```python
from build123d import *

# Parameters (mm, degrees)
MODEL_R             = 2.75
MODEL_R_2           = 1.524
MODEL_R_3           = 3.57
MODEL_R_4           = 3
MODEL_R_5           = 1.75
MODEL_R_6           = 2.988685284
MODEL_R_7           = 11.25
MODEL_W             = 18.00197115
MODEL_H             = 6.02504647
MODEL_W_2           = 25.001971156
MODEL_H_2           = 6.025046469
BOSS_EXTRUDE2_DEPTH = 3


with BuildPart() as part:
    # Model → Boss-Extrude2 (new body)
    with BuildSketch(Plane.XY):
        with BuildLine():
            Line((-1558.170802496, 1596.031612088), (-1558.170802496, 1743.759047656))
            ThreePointArc((-1558.170802496, 1743.759047656), (-1559.633113999, 1747.298520787), (-1563.170804742, 1748.765139071))
            Line((-1563.170804742, 1748.765139071), (-1643.16842822, 1748.765139071))
            ThreePointArc((-1643.16842822, 1748.765139071), (-1646.706118961, 1747.298520788), (-1648.168430466, 1743.759047658))
            Line((-1648.168430466, 1743.759047658), (-1648.168430466, 1596.031606131))
            ThreePointArc((-1648.168430466, 1596.031606131), (-1646.703964372, 1592.496072226), (-1643.168430466, 1591.031606131))
            Line((-1643.168430466, 1591.031606131), (-1563.170808452, 1591.031606131))
            ThreePointArc((-1563.170808452, 1591.031606131), (-1559.63526859, 1592.496072225), (-1558.170802496, 1596.031612088))
        make_face()
        with Locations((-1573.06309524, 1605.466177477)):
            Circle(MODEL_R, mode=Mode.SUBTRACT)
        with Locations((-1573.06309524, 1625.466177477)):
            Circle(MODEL_R, mode=Mode.SUBTRACT)
        with Locations((-1633.276137722, 1605.466177477)):
            Circle(MODEL_R, mode=Mode.SUBTRACT)
        with Locations((-1633.276137722, 1625.466177477)):
            Circle(MODEL_R, mode=Mode.SUBTRACT)
        with Locations((-1564.034669062, 1605.466177486)):
            Circle(MODEL_R, mode=Mode.SUBTRACT)
        with Locations((-1642.166137722, 1605.466177477)):
            Circle(MODEL_R, mode=Mode.SUBTRACT)
        with Locations((-1564.034669062, 1625.466177486)):
            Circle(MODEL_R, mode=Mode.SUBTRACT)
        with Locations((-1642.166137722, 1625.466177477)):
            Circle(MODEL_R, mode=Mode.SUBTRACT)
        with Locations((-1564.0520997, 1593.809639733)):
            Circle(MODEL_R_2, mode=Mode.SUBTRACT)
        with Locations((-1584.028829584, 1602.080803539)):
            Circle(MODEL_R_2, mode=Mode.SUBTRACT)
        with Locations((-1642.287133262, 1593.809639733)):
            Circle(MODEL_R_2, mode=Mode.SUBTRACT)
        with Locations((-1622.310403377, 1602.080803539)):
            Circle(MODEL_R_2, mode=Mode.SUBTRACT)
        with Locations((-1564.034669062, 1679.892967716)):
            Circle(MODEL_R, mode=Mode.SUBTRACT)
        with Locations((-1564.034669062, 1659.936167716)):
            Circle(MODEL_R, mode=Mode.SUBTRACT)
        with Locations((-1642.166137722, 1679.892967726)):
            Circle(MODEL_R, mode=Mode.SUBTRACT)
        with Locations((-1642.166137722, 1659.936167726)):
            Circle(MODEL_R, mode=Mode.SUBTRACT)
        with Locations((-1633.028888044, 1669.901183151)):
            Circle(MODEL_R_3, mode=Mode.SUBTRACT)
        with Locations((-1633.027603994, 1699.99200382)):
            Circle(MODEL_R_3, mode=Mode.SUBTRACT)
        with Locations((-1633.027603994, 1639.99200382)):
            Circle(MODEL_R_3, mode=Mode.SUBTRACT)
        with Locations((-1642.168430466, 1643.881204835)):
            Circle(MODEL_R_3, mode=Mode.SUBTRACT)
        with Locations((-1642.168430466, 1696.860624835)):
            Circle(MODEL_R_3, mode=Mode.SUBTRACT)
        with Locations((-1564.170802496, 1643.881204835)):
            Circle(MODEL_R_3, mode=Mode.SUBTRACT)
        with Locations((-1573.17191871, 1669.901183151)):
            Circle(MODEL_R_3, mode=Mode.SUBTRACT)
        with Locations((-1613.166137692, 1674.864567716)):
            Circle(MODEL_R, mode=Mode.SUBTRACT)
        with Locations((-1593.100403377, 1674.880803539)):
            Circle(MODEL_R, mode=Mode.SUBTRACT)
        with Locations((-1613.077133262, 1602.064639733)):
            Circle(MODEL_R_4, mode=Mode.SUBTRACT)
        with Locations((-1593.100403377, 1602.080803539)):
            Circle(MODEL_R_4, mode=Mode.SUBTRACT)
        with Locations((-1564.170802496, 1696.860624835)):
            Circle(MODEL_R_3, mode=Mode.SUBTRACT)
        with Locations((-1613.166137692, 1664.864567716)):
            Circle(MODEL_R, mode=Mode.SUBTRACT)
        with Locations((-1618.57210033, 1609.927346224)):
            Circle(MODEL_R_5, mode=Mode.SUBTRACT)
        with Locations((-1618.625460969, 1640.924100772)):
            Circle(MODEL_R_5, mode=Mode.SUBTRACT)
        with Locations((-1593.100403377, 1664.880803539)):
            Circle(MODEL_R, mode=Mode.SUBTRACT)
        with Locations((-1573.17320276, 1699.99200382)):
            Circle(MODEL_R_3, mode=Mode.SUBTRACT)
        with Locations((-1623.370056938, 1685.360521432)):
            Circle(MODEL_R_4, mode=Mode.SUBTRACT)
        with Locations((-1582.81965611, 1685.466121434)):
            Circle(MODEL_R_6, mode=Mode.SUBTRACT)
        with Locations((-1623.370056938, 1625.360521432)):
            Circle(MODEL_R_4, mode=Mode.SUBTRACT)
        with Locations((-1582.81965611, 1625.466121434)):
            Circle(MODEL_R_6, mode=Mode.SUBTRACT)
        with Locations((-1587.603603064, 1609.952403818)):
            Circle(MODEL_R_5, mode=Mode.SUBTRACT)
        with Locations((-1587.600403377, 1640.949204131)):
            Circle(MODEL_R_5, mode=Mode.SUBTRACT)
        with Locations((-1603.100403377, 1625.452403818)):
            Circle(MODEL_R_7, mode=Mode.SUBTRACT)
        with Locations((-1573.17320276, 1639.99200382)):
            Circle(MODEL_R_3, mode=Mode.SUBTRACT)
        Polygon((-1583.977814187, 1713.92640548), (-1583.977814187, 1719.951451949), (-1568.975843031, 1719.951451949), (-1565.975843031, 1719.951451949), (-1565.975843031, 1713.92640548), (-1568.975843031, 1713.92640548), align=None, mode=Mode.SUBTRACT)
        with Locations((-1629.171788075, 1716.938928715)):
            Rectangle(MODEL_W, MODEL_H, mode=Mode.SUBTRACT)
        with Locations((-1629.171788075, 1736.938928715)):
            Rectangle(MODEL_W, MODEL_H, mode=Mode.SUBTRACT)
        Polygon((-1583.977814187, 1733.92640548), (-1583.977814187, 1739.951451949), (-1568.975843031, 1739.951451949), (-1565.975843031, 1739.951451949), (-1565.975843031, 1733.92640548), (-1568.975843031, 1733.92640548), align=None, mode=Mode.SUBTRACT)
        with Locations((-1602.671788074, 1716.938928714)):
            Rectangle(MODEL_W_2, MODEL_H_2, mode=Mode.SUBTRACT)
        with Locations((-1602.671788074, 1736.938928714)):
            Rectangle(MODEL_W_2, MODEL_H_2, mode=Mode.SUBTRACT)
        with BuildLine():
            Line((-1583.030566378, 1696.955805603), (-1583.030566378, 1696.93660548))
            ThreePointArc((-1583.030566378, 1696.93660548), (-1583.909246034, 1694.815285137), (-1586.030566378, 1693.93660548))
            Line((-1586.030566378, 1693.93660548), (-1620.030566378, 1693.93660548))
            ThreePointArc((-1620.030566378, 1693.93660548), (-1622.151886721, 1694.815285137), (-1623.030566378, 1696.93660548))
            Line((-1623.030566378, 1696.93660548), (-1623.030566378, 1696.955805603))
            ThreePointArc((-1623.030566378, 1696.955805603), (-1622.151886721, 1699.077125947), (-1620.030566378, 1699.955805603))
            Line((-1620.030566378, 1699.955805603), (-1586.030566378, 1699.955805603))
            ThreePointArc((-1586.030566378, 1699.955805603), (-1583.909246034, 1699.077125947), (-1583.030566378, 1696.955805603))
        make_face(mode=Mode.SUBTRACT)
    extrude(amount=BOSS_EXTRUDE2_DEPTH)


solid = part.part
```
Source: CAD feature listing. Evaluate the final solid. Frame: model axes, mm. Coordinates: 2 decimals unless noted, no trailing zeros. Order: outer loops, then holes, each group sorted by start corner. A loop starts at its lowest first (then second) coordinate and runs counter-clockwise, first axis right, second up. Notation, with made-up numbers: M 80,48 L 88,48 A11 cw 88,62 Z; hole C -37,35 d8. An arc over 180 degrees is marked long. Write each question's results on one line, items separated by ' | '. Start each with the question number.
1) Section query A-A (x = -1601.5). Return the cut outline in (y, z), plus the area to 3 significant figures.
2) Section query B-B (x = -1634.5). Give the number of separate pieces and of enclosed holes in the cut face, plus the area to 3 significant figures.
3) Draft query along Y for faces 1 (the face through (-1575, 1713.926, 1)), 2 (the face through (-1633.803, 1666.416, 1.479)). Return one class per face: released by +Y, released by -Y, zero draft, split by the parting line, or undercut.
4) Line query: line 1 (Y direction, x = -1579.5, z = 1.85); line 2 (Y direction, x = -1604, z = 1.9); line 3 (X direction, y = 1717.5, z = 2.4). Output: solid intervals per line, ascending. Write a range as from..to.
Answers:
1) outline: M 1591.03,0 L 1614.32,0 L 1614.32,3 L 1591.03,3 Z; M 1636.59,0 L 1693.94,0 L 1693.94,3 L 1636.59,3 Z; M 1699.96,0 L 1713.93,0 L 1713.93,3 L 1699.96,3 Z; M 1719.95,0 L 1733.93,0 L 1733.93,3 L 1719.95,3 Z; M 1739.95,0 L 1748.77,0 L 1748.77,3 L 1739.95,3 Z | area: 352 mm^2
2) separate pieces: 8 | enclosed holes: 0 | area: 349 mm^2
3) face 1: undercut | face 2: undercut
4) line 1: y = 1591.03..1713.93, 1719.95..1733.93, 1739.95..1748.77 | line 2: y = 1591.03..1614.24, 1636.67..1693.94, 1699.96..1713.93, 1719.95..1733.93, 1739.95..1748.77 | line 3: x = -1648.17..-1638.17, -1620.17..-1615.17, -1590.17..-1583.98, -1565.98..-1558.17
